```python
from build123d import *

# Parameters (mm, degrees)
BOSS_EXTRUDE1_DEPTH      = 31.5
SKETCH3_R                = 5
CUT_EXTRUDE1_DEPTH       = 32
SKETCH3_3_R              = 5
CUT_EXTRUDE2_DEPTH       = 7
SKETCH3_5_R              = 8.5
CUT_EXTRUDE3_DEPTH       = 32
CUT_EXTRUDE4_DEPTH       = 32
SKETCH4_R                = 12.5
CUT_EXTRUDE5_DEPTH       = 14
SKETCH5_R                = 17.5
SKETCH5_R_2              = 11
BOSS_EXTRUDE2_DEPTH      = 14
BOSS_EXTRUDE2_DEPTH_BACK = 9
BOSS_EXTRUDE4_DEPTH      = 10
BOSS_EXTRUDE4_DEPTH_BACK = 4
FILLET1_R                = 5


with BuildPart() as part:
    # Sketch1 → Boss-Extrude1 (new body, symmetric)
    with BuildSketch(Plane.XY):
        Polygon((-73, -31), (67, -31), (67, 0), (-46, 0), (-46, -17), (-73, -17), align=None)
    extrude(amount=BOSS_EXTRUDE1_DEPTH, both=True)

    # Sketch3 → Cut-Extrude1 (cut, through all)
    with BuildSketch(Plane(origin=(0, 0, 0), x_dir=(1, 0, 0), z_dir=(0, 1, 0))):
        with Locations((41, -15.5)):
            Circle(SKETCH3_R)
    extrude(amount=-CUT_EXTRUDE1_DEPTH, mode=Mode.SUBTRACT)

    # Sketch3_3 → Cut-Extrude2 (cut)
    with BuildSketch(Plane(origin=(0, 0, 0), x_dir=(1, 0, 0), z_dir=(0, 1, 0))):
        with BuildLine():
            Line((41, -24.5), (67, -24.5))
            Line((67, -24.5), (67, -6.5))
            Line((67, -6.5), (41, -6.5))
            ThreePointArc((41, -6.5), (32, -15.5), (41, -24.5))
        make_face()
        with Locations((41, -15.5)):
            Circle(SKETCH3_3_R, mode=Mode.SUBTRACT)
    extrude(amount=-CUT_EXTRUDE2_DEPTH, mode=Mode.SUBTRACT)

    # Sketch3_5 → Cut-Extrude3 (cut, through all)
    with BuildSketch(Plane(origin=(0, 0, 0), x_dir=(1, 0, 0), z_dir=(0, 1, 0))):
        with Locations((-31, 15.5)):
            Circle(SKETCH3_5_R)
        with Locations((-31, -15.5)):
            Circle(SKETCH3_5_R)
    extrude(amount=-CUT_EXTRUDE3_DEPTH, mode=Mode.SUBTRACT)

    # Sketch3_6 → Cut-Extrude4 (cut, through all)
    with BuildSketch(Plane(origin=(0, 0, 0), x_dir=(1, 0, 0), z_dir=(0, 1, 0))):
        with BuildLine():
            Line((-68, 12.5), (-68, -12.5))
            ThreePointArc((-68, -12.5), (-59.5, -21), (-51, -12.5))
            Line((-51, -12.5), (-51, 12.5))
            ThreePointArc((-51, 12.5), (-59.5, 21), (-68, 12.5))
        make_face()
    extrude(amount=-CUT_EXTRUDE4_DEPTH, mode=Mode.SUBTRACT)

    # Sketch4 → Cut-Extrude5 (cut)
    with BuildSketch(Plane.XZ.offset(31)):
        with Locations((-31, 15.5)):
            Circle(SKETCH4_R)
        with Locations((-31, -15.5)):
            Circle(SKETCH4_R)
    extrude(amount=-CUT_EXTRUDE5_DEPTH, mode=Mode.SUBTRACT)



with BuildPart() as body_2:
    # Sketch5 → Boss-Extrude2 (new body, two sides)
    with BuildSketch(Plane(origin=(4, 0, 0), x_dir=(0, 0, -1), z_dir=(1, 0, 0))) as boss_extrude2_sk:
        with Locations((0, 35)):
            Circle(SKETCH5_R)
        with Locations((0, 35)):
            Circle(SKETCH5_R_2, mode=Mode.SUBTRACT)
    extrude(amount=BOSS_EXTRUDE2_DEPTH)
    extrude(boss_extrude2_sk.sketch, amount=-BOSS_EXTRUDE2_DEPTH_BACK)


with BuildPart() as part_1:
    add(part.part)

    add(body_2.part)  # Boss-Extrude4 merges body 2
    # Sketch5_6 → Boss-Extrude4 (add, two sides)
    with BuildSketch(Plane(origin=(4, 0, 0), x_dir=(0, 0, -1), z_dir=(1, 0, 0))) as boss_extrude4_sk:
        with BuildLine():
            Line((-15.5, 0), (15.5, 0))
            Line((15.5, 0), (15.5, 26.875961595))
            ThreePointArc((15.5, 26.875961595), (0, 17.5), (-15.5, 26.875961595))
            Line((-15.5, 26.875961595), (-15.5, 0))
        make_face()
    extrude(amount=BOSS_EXTRUDE4_DEPTH)
    extrude(boss_extrude4_sk.sketch, amount=-BOSS_EXTRUDE4_DEPTH_BACK)

    # Fillet1
    fillet1_edges = [part_1.edges().sort_by_distance(p)[0] for p in [
        (0, 0, 0),
        (14, 0, 0),
    ]]
    fillet(fillet1_edges, radius=FILLET1_R)


solid = part_1.part
```
Can you work these out from the model? Positions are in its coordinate system, mm. A direction names the side the tool comes from. Coordinates: 2 decimals unless noted, no trailing zeros. Loops run counter-clockwise (first coordinate to the right, second up) from the corner with the lowest first, then second, coordinate; pieces in that order, holes last. Notation, with made-up numbers: M 78.25,56 L 133.25,56 A17 cw 133.25,87 Z; hole C 23,-13.75 d10. An arc over 180 degrees is marked long. Put each result on its own line as item: value. Start each with the question number.
(1) We'd pull the mould along Y, two halves only. Please class faces 5 (the face through (-68.3, -17, 0.4)), 6 (the face through (-41, -24, -23)), 7 (the face through (-28, -17, -24)), 8 (the face through (-2, 1, 0)): +Y half, -Y half, draft (parallel to the pull), parting line (faces both ways), or undercut.
(2) Imagine slicing it at C-C on z = -9. Give the number of separate pieces and of enclosed holes in the cut face, and give its area (3 significant figures).
(3) Which directions (+Z, -Z, +X, -X, +Y, -Y) give clear straight access to the entire face, cutting with the end or side of a thin tool? Please do faces 1 (the face through (-28, -17, 7)), 2 (the face through (54, -3, 24.5)), 3 (the face through (-59.313, -23.902, -20.998)), 4 (the face through (-5, 43, -8)).
(4) Imagine slicing it at A-A on x = -59.5. List the corners of the cut face in (y, z) for me.
(5) I need wall thicknesses on probe 1 along X at (y, z) = (-8.25, 15.5); probe 2 along Z at (x, y) = (-31, -3.75); probe 3 along Z at (x, y) = (-31, -24). Which ranges of each line are inside material? Lowest first, please.
(6) Imagine slicing it at D-D on x = 49. List the corners of the cut face in (y, z) for me, and give its area (3 significant figures).
(7) Will these pins go through, and if not, where does the flat tip stop? pin 1 Ø5.5 at (x, z) = (49, 16) entering from +Y; pin 2 Ø8 at (x, z) = (16.5, -7) entering from +Y; pin 3 Ø17.5 at (y, z) = (29.5, -4.5) entering from -X.
(8) Imagine slicing it at B-B on y = -23.5. List the corners of the cut face in (x, z) for me.
Worked answers:
1. face 5: +Y half
1. face 6: draft
1. face 7: -Y half
1. face 8: undercut
2. separate pieces: 4
2. enclosed holes: 0
2. area: 3,850 mm2
3. face 1: -Y
3. face 2: +X, +Y
3. face 3: +Y, -Y
3. face 4: +Z, -Z, -X, +Y
4. outline: M -31,-31.5 L -17,-31.5 L -17,-21 L -31,-21 Z; M -31,21 L -17,21 L -17,31.5 L -31,31.5 Z
5. probe 1: x = -46 to -39.5, -22.5 to 36, 46 to 67
5. probe 2: z = -31.5 to -24, -7 to 7, 24 to 31.5
5. probe 3: z = -31.5 to -28, -3 to 3, 28 to 31.5
6. outline: M -31,-31.5 L 0,-31.5 L 0,6.5 L -7,6.5 L -7,24.5 L 0,24.5 L 0,31.5 L -31,31.5 Z
6. area: 1,830 mm2
7. pin 1: stops at y = -7
7. pin 2: stops at y = 52.24
7. pin 3: stops at x = -5
8. outline: M -73,-31.5 L 67,-31.5 L 67,31.5 L -73,31.5 Z; hole M -68,-12.5 A8.5 ccw -51,-12.5 L -51,12.5 A8.5 ccw -68,12.5 Z; hole C -31,-15.5 d25; hole C -31,15.5 d25; hole C 41,15.5 d10
